from build123d import *

# Parameters (mm, degrees)
CHAMFER1_SIZE = 0.5


with BuildPart() as part:
    # Sketch1 → Revolve1 (revolve)
    with BuildSketch(Plane.XY):
        with BuildLine():
            Line((18, 12), (18, 5))
            Line((18, 5), (3, 5))
            Line((3, 5), (3, 7))
            ThreePointArc((3, 7), (2.121320344, 9.121320344), (0, 10))
            Line((0, 10), (0, 15))
            Line((0, 15), (8, 15))
            Line((8, 15), (8, 12))
            ThreePointArc((8, 12), (11, 9), (14, 12))
            Line((14, 12), (18, 12))
        make_face()
    revolve(axis=Axis((0, 0, 0), (1, 0, 0)))

    # Chamfer1
    chamfer1_edges = [part.edges().sort_by_distance(p)[0] for p in [
        (0, -15, 0),
        (8, -15, 0),
    ]]
    chamfer(chamfer1_edges, length=CHAMFER1_SIZE)


solid = part.part
The model under review builds one solid part; all positions refer to its coordinate system, in mm. A direction names the side the tool comes from. Round coordinates to 2 decimals unless told otherwise and drop trailing zeros. Loops run counter-clockwise (first coordinate to the right, second up) from the corner with the lowest first, then second, coordinate; pieces in that order, holes last. Notation, with made-up numbers: (33, 55.5) -> (57, 55.5) arc R10 cw to (57, 74.5) -> close; hole circle Ø8 at (75.25, 22). An arc over 180 degrees is marked (long way). Return JSON: item names as keys, results as strings.
(1) For faces 1 (the cylindrical face through (16.03, -11.99, 0.53)), 2 (the flat face through (0, -3, 10)), list the 3-axis set-ups (+Z, -Z, +X, -X, +Y, -Y) from which the entire face can be reached by the end or side of a thin tool; tool diameter is ignored.
Solved:
{"face 1": "+X", "face 2": "+Z, -Z, -X, +Y, -Y"}
(2) Add section C-C on x = 3.75. Write out the cut boundary in (y, z).
Solved:
{"outline": "circle Ø30 at (0, 0); hole circle Ø10 at (0, 0)"}
(3) The part is to be moulded in two halves that separate along Y. For faces 3 (the flat face through (3, 2, 5)), 4 (the cylindrical face through (4.049, -14.985, 0.66)), 5 (the flat face through (8, 2, 12)), 6 (the cylindrical face through (10.4, -1.08, -4.88)), say which applies: released by +Y, released by -Y, zero draft, split by the parting line, or undercut.
Solved:
{"face 3": "undercut", "face 4": "split by the parting line", "face 5": "zero draft", "face 6": "undercut"}
(4) Add section D-D on x = 15.25. Write out the cut boundary in (y, z), plus the area to 3 significant figures.
Solved:
{"outline": "circle Ø24 at (0, 0); hole circle Ø10 at (0, 0)", "area": "374 mm2"}
(5) For line 1 (Z direction, x = 6, y = 0); line 2 (X direction, y = -5.75, z = -2.5); line 3 (Z direction, x = 1.5, y = 0.5), list the stretches that pass through material, from the lowest coordinate up.
Solved:
{"line 1": "-15 to -5, 5 to 15", "line 2": "3 to 18", "line 3": "-14.99 to -9.59, 9.59 to 14.99"}
(6) Add section A-A on z = 0. Write out the cut boundary in (x, y), plus the area to 3 significant figures.
Solved:
{"outline": "(0, -14.5) -> (0.5, -15) -> (7.5, -15) -> (8, -14.5) -> (8, -12) arc R3 cw to (14, -12) -> (18, -12) -> (18, -5) -> (3, -5) -> (3, -7) arc R3 cw to (0, -10) -> close; (0, 10) arc R3 cw to (3, 7) -> (3, 5) -> (18, 5) -> (18, 12) -> (14, 12) arc R3 cw to (8, 12) -> (8, 14.5) -> (7.5, 15) -> (0.5, 15) -> (0, 14.5) -> close", "area": "245 mm2"}
(7) For pin 1 (10 mm diameter, centred on x = 15, y = -3.5, fed in from -Z); pin 2 (5 mm diameter, centred on x = 10, y = -2.5, fed in from +Z); pin 3 (10 mm diameter, centred on x = 11.5, y = -8, fed in from -Z), all flat-tipped, find the tip position at first contact; note any pin that passes through.
Solved:
{"pin 1": "z = -12", "pin 2": "z = 14.82", "pin 3": "z = -14.14"}
